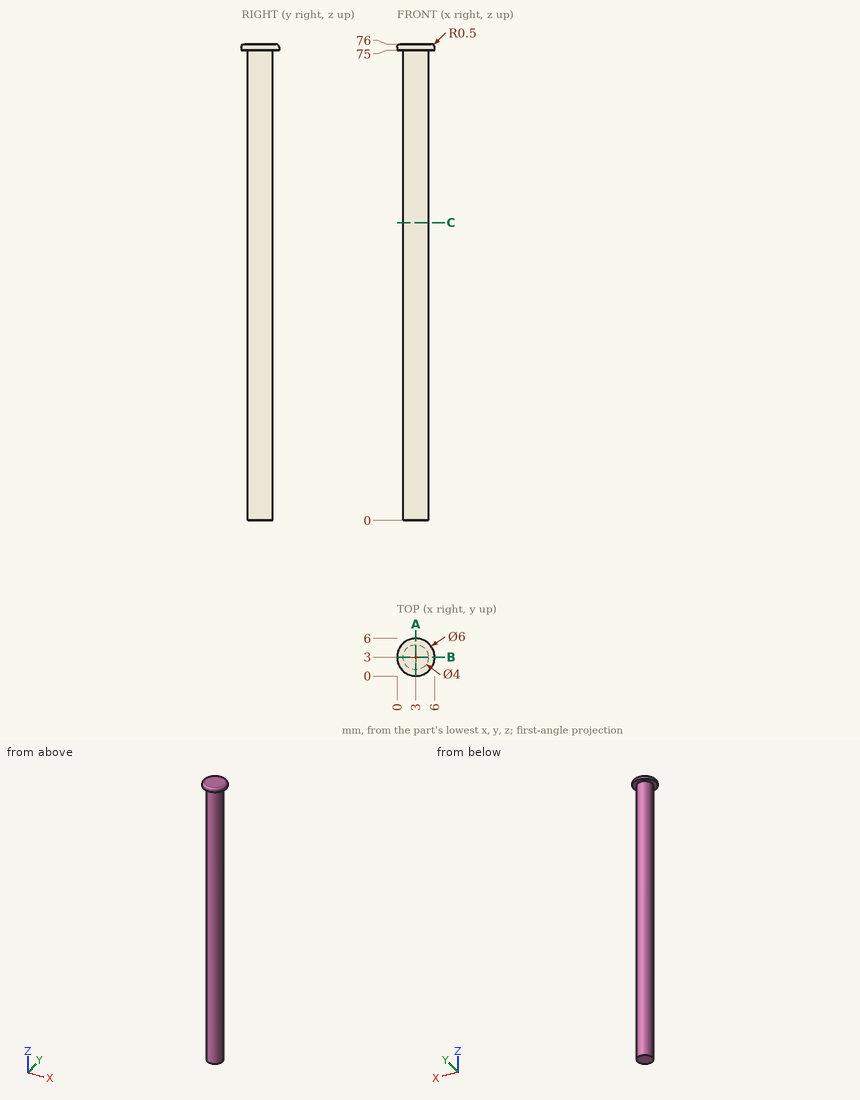
Geometry check sheet. Reference: drawing and pictorial views, mm from the part's lowest x, y, z. Coordinates: 2 decimals unless noted, no trailing zeros. Order: outer loops, then holes, each group sorted by start corner. A loop starts at its lowest first (then second) coordinate and runs counter-clockwise, first axis right, second up. Notation, with made-up numbers: M -1,-31.75 L 13,-31.75 A30 ccw 13,6.25 Z; hole C 86.5,-20 d4. An arc over 180 degrees is marked long. Write each question's results on one line, items separated by ' | '. Start each with the question number.
1. Cross-section at C-C on z = 47.5. Record the cut outline in (x, y), and give its area (3 significant figures).
2. Cross-section at A-A on x = 3. Record the cut outline in (y, z).
3. Go/stop test with flat-tipped pins: P1, Ø2, axis at x = 3.5, z = 49, coming from the +Y side; P2, Ø1.5, axis at x = 4.5, z = 29.5, coming from the +Y side; P3, Ø3, axis at y = 3.5, z = 64, coming from the +X side. Record where each tip stops, or that it passes through.
4. Material ranges on probe 1 along Y at (x, z) = (2.9, 39); probe 2 along Z at (x, y) = (5.2, 2.35); probe 3 along X at (y, z) = (3.2, 72), recorded low to high.
Checks:
1) outline: C 3,3 d4 | area: 12.6 mm²
2) outline: M 0,75 L 1,75 L 1,0 L 5,0 L 5,75 L 6,75 L 6,75.5 A0.5 ccw 5.5,76 L 0.5,76 A0.5 ccw 0,75.5 Z
3) P1: stops at y = 5 | P2: stops at y = 4.85 | P3: stops at x = 5
4) probe 1: y = 1 to 5 | probe 2: z = 75 to 76 | probe 3: x = 1.01 to 4.99
